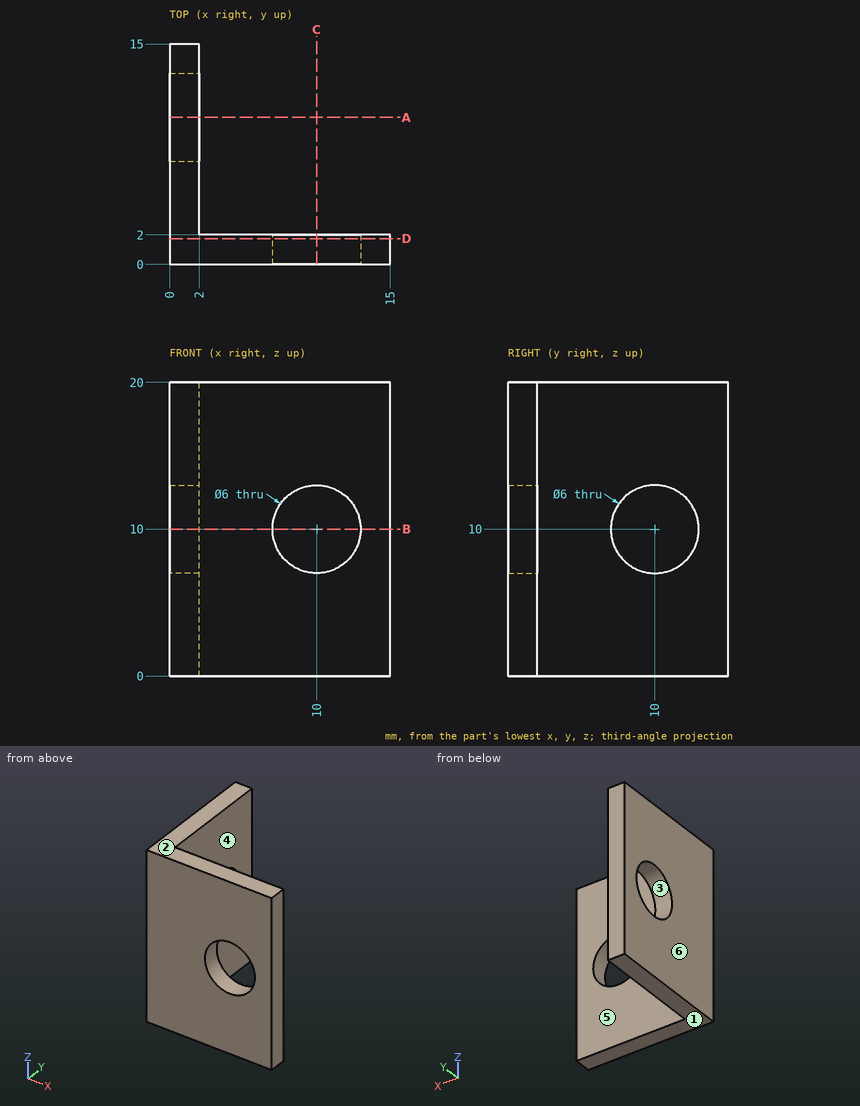
Source: three-view drawing plus pictorial views. Frame: mm from the lowest corner of the part. A direction names the side the tool comes from. Give positions to 0.01 mm unless a question says otherwise; leave off trailing zeros. Write each loop counter-clockwise with the first axis right and the second up, starting at its lowest first coordinate (ties: lowest second). Pieces come first, ordered by that corner, then holes. Notation, with made-up numbers: (68, 4) - (84, 4) arc R16 ccw to (84, 23) - close; hole circle Ø10 at (23.5, 33). An arc over 180 degrees is marked (long way). Write item = value, one per line. Start each with the question number.
Q1. Cut plane B-B, the plane z = 10. Return loops of the section in (x, y).
Q2. Material intervals for probe 1 along Z at (x, y) = (10, 0.75); probe 2 along Y at (x, z) = (1.55, 10); probe 3 along Y at (x, z) = (3.5, 16.75), sorted ascending.
Q3. Pin query (flat end, axial travel): pin 1 Ø5.5 at (y, z) = (10, 10) entering from -X; pin 2 Ø6 at (x, z) = (8, 3.5) entering from +Y; pin 3 Ø2 at (y, z) = (4.5, 15.5) entering from +X. Return the tip coordinate at first contact, or that it passes through.
Q4. Reachability of the marked faces 5 and 6 from +Z, -Z, +X, -X, +Y, -Y: full face, straight path, thin tool, end or side. Return the list, or none.
Q5. Cut plane D-D, the plane y = 1.75. Return loops of the section in (x, z).
Q6. Cut plane A-A, the plane y = 10. Return loops of the section in (x, z), then the cut area to 3 significant figures.
Q7. Draft query along Z for the marked faces 1, 2, 3 and 4. Return one class per face: +Z half, -Z half, draft (parallel to the pull), parting line (faces both ways), or undercut.
Computed values:
q1.outline = (0, 0) - (7, 0) - (7, 2) - (2, 2) - (2, 7) - (0, 7) - close; (0, 13) - (2, 13) - (2, 15) - (0, 15) - close; (13, 0) - (15, 0) - (15, 2) - (13, 2) - close
q2.probe_1 = 0 to 7, 13 to 20
q2.probe_2 = 0 to 7, 13 to 15
q2.probe_3 = 0 to 2
q3.pin_1 = through
q3.pin_2 = 2
q3.pin_3 = 2
q4.face_5 = +Z, -Z, +X, +Y
q4.face_6 = +Z, -Z, -X, +Y, -Y
q5.outline = (0, 0) - (15, 0) - (15, 20) - (0, 20) - close; hole circle Ø6 at (10, 10)
q6.outline = (0, 0) - (2, 0) - (2, 7) - (0, 7) - close; (0, 13) - (2, 13) - (2, 20) - (0, 20) - close
q6.area = 28.0 mm²
q7.face_1 = -Z half
q7.face_2 = +Z half
q7.face_3 = undercut
q7.face_4 = draft
